```python
from build123d import *

# Parameters (mm, degrees)
ESBO_O1_R                     = 35
ESBO_O1_R_2                   = 32.5
RESSALTO_EXTRUS_O1_DEPTH      = 8
RESSALTO_EXTRUS_O2_START      = -3
ESBO_O2_R                     = 32.5
RESSALTO_EXTRUS_O2_DEPTH      = 3
ESBO_O3_R                     = 2.5
CORTE_EXTRUS_O1_DEPTH         = 3
RESSALTO_EXTRUS_O3_DEPTH      = 5
RESSALTO_EXTRUS_O3_DEPTH_BACK = 3
ESBO_O4_R                     = 37
ESBO_O4_R_2                   = 35
ESBO_O5_W                     = 1.8
ESBO_O5_H                     = 3
ESBO_O6_R                     = 12.55
RESSALTO_EXTRUS_O4_DEPTH      = 5
CORTE_EXTRUS_O2_DEPTH         = 53.933921071
CORTE_EXTRUS_O2_DEPTH_BACK    = 53.933921071
ESBO_O7_R                     = 7.55
RESSALTO_EXTRUS_O5_START      = -8
ESBO_O8_R                     = 37
ESBO_O8_R_2                   = 32.5
RESSALTO_EXTRUS_O5_DEPTH      = 8
ESBO_O9_R                     = 37
ESBO_O9_R_2                   = 33.5
CORTE_EXTRUS_O8_DEPTH         = 1.5
CORTE_EXTRUS_O9_START         = -1.5
ESBO_O12_R                    = 37
ESBO_O12_R_2                  = 33.5
CORTE_EXTRUS_O9_DEPTH         = 1.5
CORTE_EXTRUS_O10_START        = -10
ESBO_O13_R                    = 37
ESBO_O13_R_2                  = 36
CORTE_EXTRUS_O10_DEPTH        = 10
ESBO_O14_R                    = 37
ESBO_O14_R_2                  = 36
RESSALTO_EXTRUS_O6_DEPTH      = 5
ESBO_O15_R                    = 12.55
CORTE_EXTRUS_O11_DEPTH        = 53.933921071
ESBO_O16_R                    = 12.55
RESSALTO_EXTRUS_O7_DEPTH      = 3
ESBO_O17_R                    = 10
RESSALTO_EXTRUS_O8_DEPTH      = 16
ESBO_O18_R                    = 3.3
CORTE_EXTRUS_O12_DEPTH        = 16
ESBO_O19_W                    = 5.95
ESBO_O19_H                    = 2.65
CORTE_EXTRUS_O13_DEPTH        = 8
ESBO_O23_R                    = 37
ESBO_O23_R_2                  = 36
CORTE_EXTRUS_O15_DEPTH        = 54.798234172
ESBO_O24_R                    = 3.3
RESSALTO_EXTRUS_O9_DEPTH      = 11
CORTE_EXTRUS_O14_DEPTH        = 56.88103435
CORTE_EXTRUS_O14_DEPTH_BACK   = 56.88103435
ESBO_O21_R                    = 1.65


with BuildPart() as part:
    # Esboço1 → Ressalto-extrusão1 (new body)
    with BuildSketch(Plane.XY):
        Circle(ESBO_O1_R)
        Circle(ESBO_O1_R_2, mode=Mode.SUBTRACT)
    extrude(amount=RESSALTO_EXTRUS_O1_DEPTH)

    # Esboço2 → Ressalto-extrusão2 (add)
    with BuildSketch(Plane.XY.offset(8).offset(RESSALTO_EXTRUS_O2_START)):
        Circle(ESBO_O2_R)
    extrude(amount=RESSALTO_EXTRUS_O2_DEPTH)

    # Esboço3 → Corte-extrusão1 (cut)
    with BuildSketch(Plane.XY.offset(8)):
        Circle(ESBO_O3_R)
    extrude(amount=-CORTE_EXTRUS_O1_DEPTH, mode=Mode.SUBTRACT)

    # Esboço4 → Ressalto-extrusão3 (add, two sides: drawn at the far end of the back side and taken through both)
    with BuildSketch(Plane(origin=(0, 0, 5), x_dir=(-1, 0, 0), z_dir=(0, 0, -1)).offset(-RESSALTO_EXTRUS_O3_DEPTH_BACK)):
        Circle(ESBO_O4_R)
        Circle(ESBO_O4_R_2, mode=Mode.SUBTRACT)
    extrude(amount=RESSALTO_EXTRUS_O3_DEPTH + RESSALTO_EXTRUS_O3_DEPTH_BACK)

    # Esboço5 → Corte-Revolução1 (revolve, cut)
    with BuildSketch(Plane(origin=(0, 0, 0), x_dir=(1, 0, 0), z_dir=(0, 1, 0))):
        with Locations((-36.1, -2.5)):
            Rectangle(ESBO_O5_W, ESBO_O5_H)
        with Locations((-36.1, -5.5)):
            Rectangle(ESBO_O5_W, ESBO_O5_H)
    revolve(axis=Axis((0, 0, 8), (0, 0, -1)), mode=Mode.SUBTRACT)

    # Esboço6 → Ressalto-extrusão4 (add)
    with BuildSketch(Plane(origin=(0, 0, 5), x_dir=(-1, 0, 0), z_dir=(0, 0, -1))):
        with Locations(Location((0, 0, 0), (0, 0, 180))):
            Circle(ESBO_O6_R)
    extrude(amount=RESSALTO_EXTRUS_O4_DEPTH)

    # Esboço7 → Corte-extrusão2 (cut, two sides: drawn at the far end of the back side and taken through both)
    with BuildSketch(Plane(origin=(0, 0, 0), x_dir=(-1, 0, 0), z_dir=(0, 0, -1)).offset(-CORTE_EXTRUS_O2_DEPTH_BACK)):
        Circle(ESBO_O7_R)
    extrude(amount=CORTE_EXTRUS_O2_DEPTH + CORTE_EXTRUS_O2_DEPTH_BACK, mode=Mode.SUBTRACT)

    # Esboço8 → Ressalto-extrusão5 (add)
    with BuildSketch(Plane.XY.offset(8).offset(RESSALTO_EXTRUS_O5_START)):
        with Locations(Location((0, 0, 0), (0, 0, 180))):
            Circle(ESBO_O8_R)
        Circle(ESBO_O8_R_2, mode=Mode.SUBTRACT)
    extrude(amount=RESSALTO_EXTRUS_O5_DEPTH)

    # Esboço9 → Corte-extrusão8 (cut)
    with BuildSketch(Plane.XY.offset(8)):
        with Locations(Location((0, 0, 0), (0, 0, 180))):
            Circle(ESBO_O9_R)
        Circle(ESBO_O9_R_2, mode=Mode.SUBTRACT)
    extrude(amount=-CORTE_EXTRUS_O8_DEPTH, mode=Mode.SUBTRACT)

    # Esboço12 → Corte-extrusão9 (cut)
    with BuildSketch(Plane(origin=(0, 0, 0), x_dir=(-1, 0, 0), z_dir=(0, 0, -1)).offset(CORTE_EXTRUS_O9_START)):
        Circle(ESBO_O12_R)
        with Locations(Location((0, 0, 0), (0, 0, 180))):
            Circle(ESBO_O12_R_2, mode=Mode.SUBTRACT)
    extrude(amount=CORTE_EXTRUS_O9_DEPTH, mode=Mode.SUBTRACT)

    # Esboço13 → Corte-extrusão10 (cut)
    with BuildSketch(Plane(origin=(0, 0, 1.5), x_dir=(-1, 0, 0), z_dir=(0, 0, -1)).offset(CORTE_EXTRUS_O10_START)):
        Circle(ESBO_O13_R)
        Circle(ESBO_O13_R_2, mode=Mode.SUBTRACT)
    extrude(amount=CORTE_EXTRUS_O10_DEPTH, mode=Mode.SUBTRACT)

    # Esboço14 → Ressalto-extrusão6 (add)
    with BuildSketch(Plane.XY.offset(6.5)):
        Circle(ESBO_O14_R)
        Circle(ESBO_O14_R_2, mode=Mode.SUBTRACT)
    extrude(amount=-RESSALTO_EXTRUS_O6_DEPTH)

    # Esboço15 → Corte-extrusão11 (cut, through all)
    with BuildSketch(Plane(origin=(0, 0, 0), x_dir=(-1, 0, 0), z_dir=(0, 0, -1))):
        Circle(ESBO_O15_R)
    extrude(amount=-CORTE_EXTRUS_O11_DEPTH, mode=Mode.SUBTRACT)

    # Esboço16 → Ressalto-extrusão7 (add, through all)
    with BuildSketch(Plane(origin=(0, 0, 5), x_dir=(-1, 0, 0), z_dir=(0, 0, -1))):
        Circle(ESBO_O16_R)
    extrude(amount=-RESSALTO_EXTRUS_O7_DEPTH)

    # Esboço17 → Ressalto-extrusão8 (add)
    with BuildSketch(Plane(origin=(0, 0, 5), x_dir=(-1, 0, 0), z_dir=(0, 0, -1))):
        with Locations(Location((0, 0, 0), (0, 0, 180))):
            Circle(ESBO_O17_R)
    extrude(amount=RESSALTO_EXTRUS_O8_DEPTH)

    # Esboço18 → Corte-extrusão12 (cut)
    with BuildSketch(Plane(origin=(0, 0, -11), x_dir=(-1, 0, 0), z_dir=(0, 0, -1))):
        Circle(ESBO_O18_R)
    extrude(amount=-CORTE_EXTRUS_O12_DEPTH, mode=Mode.SUBTRACT)

    # Esboço19 → Corte-extrusão13 (cut)
    with BuildSketch(Plane(origin=(0, 0, -11), x_dir=(-1, 0, 0), z_dir=(0, 0, -1))):
        with Locations((0, -6.625)):
            Rectangle(ESBO_O19_W, ESBO_O19_H)
        with Locations((0, 6.625)):
            Rectangle(ESBO_O19_W, ESBO_O19_H)
    extrude(amount=-CORTE_EXTRUS_O13_DEPTH, mode=Mode.SUBTRACT)

    # Esboço23 → Corte-extrusão15 (cut, through all)
    with BuildSketch(Plane(origin=(0, 0, 1.5), x_dir=(-1, 0, 0), z_dir=(0, 0, -1))):
        Circle(ESBO_O23_R)
        Circle(ESBO_O23_R_2, mode=Mode.SUBTRACT)
    extrude(amount=-CORTE_EXTRUS_O15_DEPTH, mode=Mode.SUBTRACT)

    # Esboço24 → Ressalto-extrusão9 (add)
    with BuildSketch(Plane(origin=(0, 0, -11), x_dir=(-1, 0, 0), z_dir=(0, 0, -1))):
        Circle(ESBO_O24_R)
        with BuildLine():
            Line((-1.229837388, 1.1), (1.229837388, 1.1))
            ThreePointArc((1.229837388, 1.1), (0, -1.65), (-1.229837388, 1.1))
        make_face(mode=Mode.SUBTRACT)
    extrude(amount=-RESSALTO_EXTRUS_O9_DEPTH)

    # Esboço21 → Corte-extrusão14 (cut, two sides: drawn at the far end of the back side and taken through both)
    with BuildSketch(Plane(origin=(0, 5.3, 0), x_dir=(1, 0, 0), z_dir=(0, 1, 0)).offset(-CORTE_EXTRUS_O14_DEPTH_BACK)):
        with Locations((0, 6.85)):
            Circle(ESBO_O21_R)
    extrude(amount=CORTE_EXTRUS_O14_DEPTH + CORTE_EXTRUS_O14_DEPTH_BACK, mode=Mode.SUBTRACT)


solid = part.part
```
Read the model definition and answer for the solid it produces. Units are mm, in the model's axes. A direction names the side the tool comes from. Give positions to 0.01 mm unless a question says otherwise; leave off trailing zeros. Write each loop counter-clockwise with the first axis right and the second up, starting at its lowest first coordinate (ties: lowest second). Pieces come first, ordered by that corner, then holes. Notation, with made-up numbers: (87.25, 45.25) -> (97.25, 45.25) arc R20 ccw to (97.25, 84.25) -> close; hole circle Ø5 at (-15.5, 61.25). An arc over 180 degrees is marked (long way). Answer in a Markdown table with one row per item.
1) Section B-B on x = 0 is taken. Count the separate pieces of the cut face and the enclosed holes in it, plus the area to 3 significant figures.
Results list:
| item | result |
|---|---|
| separate pieces | 5 |
| enclosed holes | 0 |
| area | 411 mm^2 |
2) Determine the mould class of faces 4 (the cylindrical face through (31, 9.76, 2.46)), 5 (the cylindrical face through (30.945, 12.831, 0.76)), 6 (the flat face through (24, -24, 1.5)) for opening direction Y: released by +Y, released by -Y, zero draft, split by the parting line, or undercut.
Results list:
| item | result |
|---|---|
| face 4 | undercut |
| face 5 | split by the parting line |
| face 6 | zero draft |
3) Straight lines are drawn through the part: line 1 (Z direction, x = 0, y = 2); line 2 (Z direction, x = 0, y = 3.4); line 3 (Y direction, x = 1, z = 0.5). For each, find the intervals that lie inside material, in ascending order. Write a range as [from, to].
Results list:
| item | result |
|---|---|
| line 1 | [-11, -8.5], [-5.2, 0], [5, 8] |
| line 2 | [-11, -8.5], [-5.2, 8] |
| line 3 | [-33.49, -32.48], [-9.95, -3.14], [3.14, 9.95], [32.48, 33.49] |
4) Section A-A on z = -9.75 is taken. Give the vertices of the cut face in (x, y) (3 decimals).
Results list:
| item | result |
|---|---|
| outline | circle Ø20 at (0, 0); hole (-2.975, -7.95) -> (2.975, -7.95) -> (2.975, -5.3) -> (-2.975, -5.3) -> close; hole (-2.975, 5.3) -> (2.975, 5.3) -> (2.975, 7.95) -> (-2.975, 7.95) -> close; hole (-1.23, 1.1) arc R1.65 ccw (long way) to (1.23, 1.1) -> close |
5) A tool of negligible diameter and unlimited length cuts with its end or side. For faces 1 (the cylindrical face through (2.43, 2.23, 2.46)), 2 (the cylindrical face through (-7.262, -32.703, 7.26)), 3 (the flat face through (0, 1.1, -9)), from which of +Z, -Z, +X, -X, +Y, -Y can it reach the whole face along a straight path? Write none if from no direction.
Results list:
| item | result |
|---|---|
| face 1 | none |
| face 2 | +Z |
| face 3 | -Z |
6) Each of these flat-tipped pins is pushed along its axis until it touches: pin 1 Ø0.8 at (y, z) = (6.5, -5.5) entering from -X; pin 2 Ø2.5 at (x, z) = (0, -6.85) entering from +Y; pin 3 Ø6.5 at (x, z) = (-1.5, -6) entering from +Y; pin 4 Ø8 at (y, z) = (9, 4.5) entering from -X. Where does it stop, or does it pass through?
Results list:
| item | result |
|---|---|
| pin 1 | x = -7.92 |
| pin 2 | through |
| pin 3 | y = 10 |
| pin 4 | x = -35.65 |
7) Section D-D on x = -18 is taken. Give the vertices of the cut face in (y, z).
Results list:
| item | result |
|---|---|
| outline | (-31.18, 1.5) -> (-28.25, 1.5) -> (-28.25, 0) -> (-27.06, 0) -> (-27.06, 5) -> (27.06, 5) -> (27.06, 0) -> (28.25, 0) -> (28.25, 1.5) -> (31.18, 1.5) -> (31.18, 6.5) -> (28.25, 6.5) -> (28.25, 8) -> (-28.25, 8) -> (-28.25, 6.5) -> (-31.18, 6.5) -> close |
8) Section C-C on y = -19.5 is taken. Give the vertices of the cut face in (x, z).
Results list:
| item | result |
|---|---|
| outline | (-30.26, 1.5) -> (-27.24, 1.5) -> (-27.24, 0) -> (-26, 0) -> (-26, 5) -> (26, 5) -> (26, 0) -> (27.24, 0) -> (27.24, 1.5) -> (30.26, 1.5) -> (30.26, 6.5) -> (27.24, 6.5) -> (27.24, 8) -> (-27.24, 8) -> (-27.24, 6.5) -> (-30.26, 6.5) -> close |
